Verification items for the finished model (mm, model axes). A direction names the side the tool comes from. Give positions to 0.01 mm unless a question says otherwise; leave off trailing zeros. Order: outer loops, then holes, each group sorted by start corner. A loop starts at its lowest first (then second) coordinate and runs counter-clockwise, first axis right, second up. Notation, with made-up numbers: (62, 29) -> (77, 29) arc R30 cw to (77, 61) -> close; hole circle Ø4 at (84.5, -9). An arc over 180 degrees is marked (long way). Return JSON: item names as keys, results as strings. Group by question number.
(1) Cross-section at D-D on y = 3. Enter the section's corners in (x, z), then the cut area to 4 significant figures.
(2) Cross-section at C-C on x = 74.3. Enter the section's corners in (y, z), then the cut area to 3 significant figures.
(3) Cross-section at A-A on y = 54.1. Enter the section's corners in (x, z).
(4) Cross-section at B-B on z = 8.75. Enter the section's corners in (x, y), then the cut area to 3 significant figures.
(5) Release check for a two-part mould opening along X. For faces 6 (the face through (54, 0, 1)), 7 (the face through (106, 3, 1)), 8 (the face through (110.5, 35, 6)) record: pulls with the +X half, pulls with the -X half, needs draft (parallel to the pull), parting line crosses it, or undercut.
(6) Tool access check on faces 1 (the face through (25, 5, 9)), 2 (the face through (11, 78, 8)), 3 (the face through (100.5, 23, 10)), 4 (the face through (105, 38, 10)), 5 (the face through (104, 51, 13)). Record the directions out of +Z, -Z, +X, -X, +Y, -Y that give a thin tool (end or side, any length) a straight path to the whole face; none if there is none.
(7) Thickness scan on line 1 along Y through (x, z) = (105.5, 8.25); line 2 along Y through (x, z) = (2.8, 0.8); line 3 along X through (y, z) = (82, 5.75). Record the ranges inside material, lowest first.
(8) Depth check by flat-ended pin: pin 1 Ø8 at (x, y) = (81, 16.5) entering from +Z; pin 2 Ø8 at (y, z) = (47, 10.5) entering from +X; pin 3 Ø2.5 at (x, y) = (74.3, 54.1) entering from +Z; pin 4 Ø3.5 at (y, z) = (-2, 7.5) entering from +X. Enter the tip coordinate at first touch or a pass-through.
Autodesk Inventor part; units mm, degrees
ref_plane "YZ Plane" through (0, 0, 0) normal (1, 0, 0) x (0, 1, 0)
ref_plane "XZ Plane" through (0, 0, 0) normal (0, 1, 0) x (-1, 0, 0)
ref_plane "XY Plane" through (0, 0, 0) normal (0, 0, 1) x (1, 0, 0)
sketch "Sketch1" plane through (0, 0, 0) normal (0, 0, 1) x (1, 0, 0)
  line L0 (0, 0) -> (110.5, 0)
  line L1 (110.5, 0) -> (110.5, 91.3)
  line L2 (110.5, 91.3) -> (0, 91.3)
  line L3 (0, 91.3) -> (0, 0)
  circle A0 centre (2.8, 3) radius 1.5
  circle A1 centre (74.3, 54.1) radius 1.5
  circle A2 centre (3.6, 88.5) radius 1.5
  circle A3 centre (107.5, 3) radius 1.5
  circle A4 centre (107.8, 89) radius 1.5
  dimension "d0" = 110.5
  dimension "d1" = 91.3
  dimension "d2" = 3
  dimension "d3" = 3
  dimension "d4" = 3
  dimension "d5" = 3
  dimension "d6" = 3
  dimension "d7" = 2.8
  dimension "d8" = 3
  dimension "d9" = 3.6
  dimension "d10" = 88.5
  dimension "d11" = 74.3
  dimension "d12" = 54.1
  dimension "d13" = 107.5
  dimension "d14" = 3
  dimension "d15" = 89
  dimension "d16" = 107.8
extrude "Extrusion1" add sketch "Sketch1" along normal blind 3
sketch "Sketch2" plane through (0, 0, 3) normal (0, 0, 1) x (1, 0, 0)
  line L0 (110.5, 91.3) -> (0, 91.3)
  line L1 (0, 91.3) -> (0, 0)
  line L2 (0, 83.3) -> (10, 83.3)
  line L3 (10, 83.3) -> (10, 23.3)
  line L4 (10, 23.3) -> (0, 23.3)
  line L5 (0, 23.3) -> (0, 83.3)
  dimension "d19" = 10
  dimension "d20" = 60
  dimension "d21" = 8
extrude "Extrusion2" add sketch "Sketch2" along normal blind 14
sketch "Sketch3" plane through (0, 0, 3) normal (0, 0, 1) x (1, 0, 0)
  line L0 (110.5, 0) -> (110.5, 91.3)
  line L1 (110.5, 91.3) -> (0, 91.3)
  line L2 (106, 91.3) -> (11, 91.3)
  line L3 (11, 91.3) -> (11, 65.3)
  line L4 (11, 65.3) -> (106, 65.3)
  line L5 (106, 65.3) -> (106, 91.3)
  dimension "d24" = 95
  dimension "d25" = 26
  dimension "d26" = 0
  dimension "d27" = 4.5
extrude "Extrusion3" add sketch "Sketch3" along normal blind 10
sketch "Sketch4" plane through (0, 0, 3) normal (0, 0, 1) x (1, 0, 0)
  line L0 (0, 23.3) -> (0, 0)
  line L1 (0, 0) -> (110.5, 0)
  line L2 (20, 5) -> (31, 5)
  line L3 (31, 5) -> (31, -11)
  line L4 (31, -11) -> (20, -11)
  line L5 (20, -11) -> (20, 5)
  dimension "d30" = 11
  dimension "d31" = 16
  dimension "d32" = 20
  dimension "d33" = 5
extrude "Extrusion4" add sketch "Sketch4" along normal blind 12
sketch "Sketch5" plane through (0, 0, 3) normal (0, 0, 1) x (1, 0, 0)
  line L0 (31, 0) -> (110.5, 0)
  line L1 (110.5, 0) -> (110.5, 91.3)
  line L2 (110.5, 8) -> (100.5, 8)
  line L3 (100.5, 8) -> (100.5, 38)
  line L4 (100.5, 38) -> (110.5, 38)
  line L5 (110.5, 38) -> (110.5, 8)
  dimension "d36" = 10
  dimension "d37" = 30
  dimension "d38" = 8
extrude "Extrusion5" add sketch "Sketch5" along normal blind 14
sketch "Sketch6" plane through (0, 0, 3) normal (0, 0, 1) x (1, 0, 0)
  line L0 (100.5, 38) -> (110.5, 38)
  line L1 (110.5, 38) -> (110.5, 91.3)
  line L2 (100.5, 41) -> (108.5, 41)
  line L3 (108.5, 41) -> (108.5, 61)
  line L4 (108.5, 61) -> (100.5, 61)
  line L5 (100.5, 61) -> (100.5, 41)
  dimension "d41" = 8
  dimension "d42" = 2
  dimension "d43" = 3
  dimension "d44" = 20
extrude "Extrusion6" add sketch "Sketch6" along normal blind 10
properties part number "Megatronics3.0"
Verdict:
{
 "1": {"outline": "(0, 0) -> (1.3, 0) -> (1.3, 3) -> (0, 3) -> close; (4.3, 0) -> (106, 0) -> (106, 3) -> (31, 3) -> (31, 15) -> (20, 15) -> (20, 3) -> (4.3, 3) -> close; (109, 0) -> (110.5, 0) -> (110.5, 3) -> (109, 3) -> close", "area": "445.5 mm²"},
 "2": {"outline": "(0, 0) -> (52.6, 0) -> (52.6, 3) -> (0, 3) -> close; (55.6, 0) -> (91.3, 0) -> (91.3, 13) -> (65.3, 13) -> (65.3, 3) -> (55.6, 3) -> close", "area": "525 mm²"},
 "3": {"outline": "(0, 0) -> (72.8, 0) -> (72.8, 3) -> (10, 3) -> (10, 17) -> (0, 17) -> close; (75.8, 0) -> (110.5, 0) -> (110.5, 3) -> (108.5, 3) -> (108.5, 13) -> (100.5, 13) -> (100.5, 3) -> (75.8, 3) -> close"},
 "4": {"outline": "(0, 23.3) -> (10, 23.3) -> (10, 83.3) -> (0, 83.3) -> close; (11, 65.3) -> (106, 65.3) -> (106, 91.3) -> (11, 91.3) -> close; (20, -11) -> (31, -11) -> (31, 5) -> (20, 5) -> close; (100.5, 8) -> (110.5, 8) -> (110.5, 38) -> (100.5, 38) -> close; (100.5, 41) -> (108.5, 41) -> (108.5, 61) -> (100.5, 61) -> close", "area": "3,710 mm²"},
 "5": {"face 6": "needs draft", "face 7": "undercut", "face 8": "pulls with the +X half"},
 "6": {"face 1": "+Z, +X, -X", "face 2": "+Z, +Y, -Y", "face 3": "+Z, -Y", "face 4": "+Z, +X", "face 5": "+Z, +X, +Y"},
 "7": {"line 1": "8 to 38, 41 to 61, 65.3 to 91.3", "line 2": "0 to 1.5, 4.5 to 87.23, 89.77 to 91.3", "line 3": "0 to 10, 11 to 106"},
 "8": {"pin 1": "z = 3", "pin 2": "x = 108.5", "pin 3": "through", "pin 4": "x = 31"}
}
